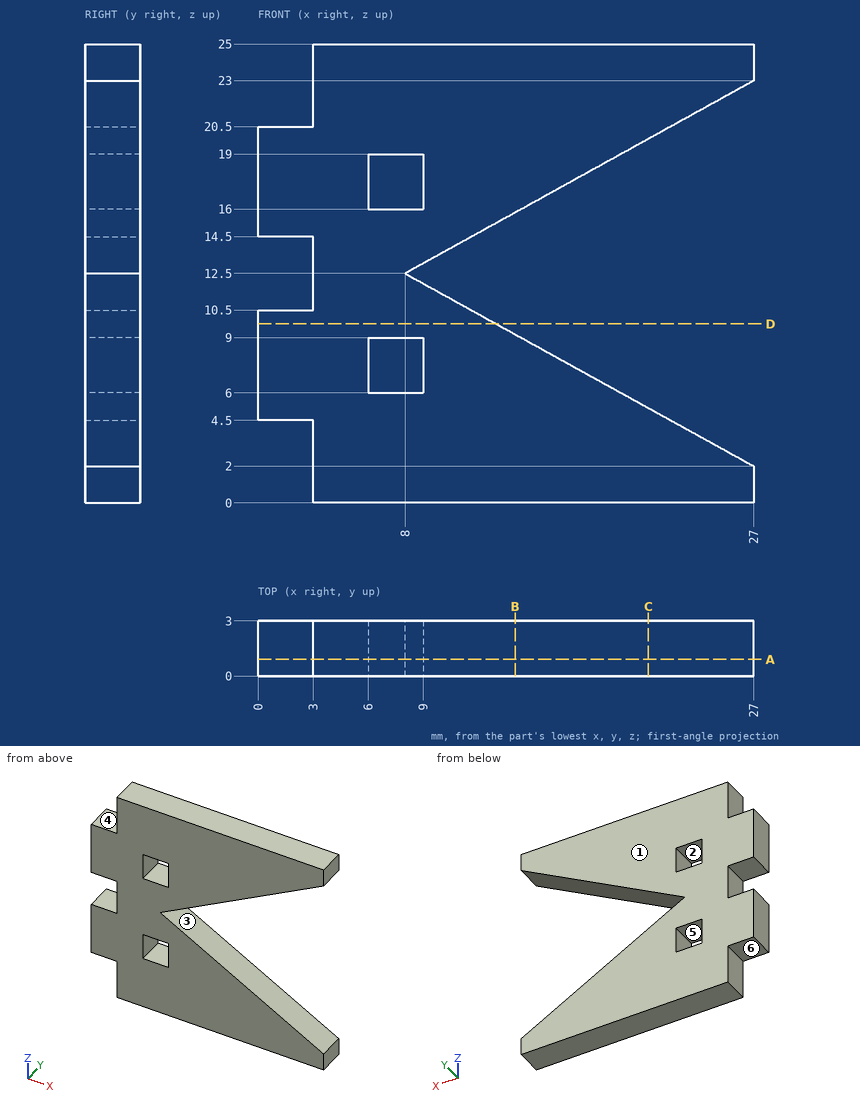
Can you work these out from the drawing? Everything is in mm from the part's minimum corner. A direction names the side the tool comes from. Coordinates: 2 decimals unless noted, no trailing zeros. Loops run counter-clockwise (first coordinate to the right, second up) from the corner with the lowest first, then second, coordinate; pieces in that order, holes last. Notation, with made-up numbers: M 25.25,74.5 L 51.25,74.5 A8 ccw 51.25,82.5 Z; hole C 62,85.25 d8. An arc over 180 degrees is marked long. Put each result on its own line as item: value. Start each with the question number.
(1) I need wall thicknesses on line 1 (Z direction, x = 8.5, y = 2.7); line 2 (Z direction, x = 2.25, y = 1.05); line 3 (Z direction, x = 12, y = 1.65). Which ranges of each line are inside material? Lowest first, please. Write a range as from..to.
(2) Will these pins go through, and if not, where does the flat tip stop? P1, Ø0.9, axis at y = 2, z = 2, coming from the -X side; P2, Ø1.5, axis at x = 1, y = 1.5, coming from the +Z side.
(3) Suppose I cut it at B-B on x = 14. Please give me the cut outline in (y, z).
(4) Suppose I cut it at A-A on y = 0.9. Please give me the cut outline in (x, z).
(5) For the marked faces 4, 5 and 6, which set-ups out of +Z, -Z, +X, -X, +Y, -Y let a thin tool reach every point of the face, with its end or its side?
(6) Suppose I cut it at C-C on x = 21.25. Please give me the cut outline in (y, z).
(7) Suppose I cut it at D-D on z = 9.75. Please give me the cut outline in (x, y), then the cut area to 3 significant figures.
(8) Thinking about a two-plate mould opening in X: for the marked faces 1, 2 and 3, which applies, pulls with the +X half, pulls with the -X half, needs draft (parallel to the pull), parting line crosses it, or undercut?
Solutions:
1. line 1: z = 0..6, 9..12.22, 12.78..16, 19..25
1. line 2: z = 4.5..10.5, 14.5..20.5
1. line 3: z = 0..10.29, 14.71..25
2. P1: stops at x = 3
2. P2: stops at z = 20.5
3. outline: M 0,0 L 3,0 L 3,9.18 L 0,9.18 Z; M 0,15.82 L 3,15.82 L 3,25 L 0,25 Z
4. outline: M 0,4.5 L 3,4.5 L 3,0 L 27,0 L 27,2 L 8,12.5 L 27,23 L 27,25 L 3,25 L 3,20.5 L 0,20.5 L 0,14.5 L 3,14.5 L 3,10.5 L 0,10.5 Z; hole M 6,6 L 9,6 L 9,9 L 6,9 Z; hole M 6,16 L 9,16 L 9,19 L 6,19 Z
5. face 4: +Z, -X, +Y, -Y
5. face 5: +Y, -Y
5. face 6: -Z, -X, +Y, -Y
6. outline: M 0,0 L 3,0 L 3,5.18 L 0,5.18 Z; M 0,19.82 L 3,19.82 L 3,25 L 0,25 Z
7. outline: M 0,0 L 12.98,0 L 12.98,3 L 0,3 Z
7. area: 38.9 mm2
8. face 1: needs draft
8. face 2: undercut
8. face 3: pulls with the +X half
